Design review of the part built by this model. Coordinates are the model's own, in mm. A direction names the side the tool comes from. Give positions to 0.01 mm unless a question says otherwise; leave off trailing zeros. Write each loop counter-clockwise with the first axis right and the second up, starting at its lowest first coordinate (ties: lowest second). Pieces come first, ordered by that corner, then holes. Notation, with made-up numbers: M 3.25,77 L 33.25,77 A14 ccw 33.25,101 Z; hole C -18,-2 d1. An arc over 180 degrees is marked long. Answer in a Markdown table with one row per item.
```python
from build123d import *

# Parameters (mm, degrees)
SKETCH001_W                 = 93
SKETCH001_H                 = 73
PAD_DEPTH                   = 10
THICKNESS_T                 = 2.5
SKETCH002_R                 = 1.7
HOLE_DEPTH                  = 25
SKETCH003_R                 = 3.7
SKETCH003_R_2               = 1.7
PAD001_DEPTH                = 2
SKETCH003_MIRRORED_2_R      = 3.7
SKETCH003_MIRRORED_2_R_2    = 1.7
PAD001_MIRRORED_2_DEPTH     = 2
SKETCH005_R                 = 1.7
POCKET_DEPTH                = 254.24889
SKETCH005_MIRRORED004_2_R   = 1.7
POCKET_MIRRORED004_2_DEPTH  = 254.24889
SKETCH006_R                 = 3.2
SKETCH006_R_2               = 2.7
PAD003_DEPTH                = 2
SKETCH006_MIRRORED006_2_R   = 3.2
SKETCH006_MIRRORED006_2_R_2 = 2.7
PAD003_MIRRORED006_2_DEPTH  = 2


with BuildPart() as part:
    # Sketch001 → Pad (new body)
    with BuildSketch(Plane.XY):
        Rectangle(SKETCH001_W, SKETCH001_H)
    extrude(amount=PAD_DEPTH)

    # Thickness
    thickness_openings = [part.faces().sort_by_distance(p)[0] for p in [
        (0, 0, 10),
    ]]
    offset(amount=THICKNESS_T, openings=thickness_openings)

    # Sketch002 → Hole (cut)
    with BuildSketch(Plane.XY):
        with Locations((-40, 30)):
            Circle(SKETCH002_R)
    extrude(amount=-HOLE_DEPTH, mode=Mode.SUBTRACT)

    # Sketch003 → Pad001 (join)
    with BuildSketch(Plane.XY):
        with Locations((-40, 30)):
            Circle(SKETCH003_R)
        with Locations((-40, 30)):
            Circle(SKETCH003_R_2, mode=Mode.SUBTRACT)
    pad001 = extrude(amount=PAD001_DEPTH)

    # Sketch003 Mirrored 2 → Pad001 Mirrored 2 (add)
    with BuildSketch(Plane(origin=(0, 0, 0), x_dir=(-1, 0, 0), z_dir=(0, 0, -1))):
        with Locations((-40, 30)):
            Circle(SKETCH003_MIRRORED_2_R)
        with Locations((-40, 30)):
            Circle(SKETCH003_MIRRORED_2_R_2, mode=Mode.SUBTRACT)
    pad001_mirrored_2 = extrude(amount=-PAD001_MIRRORED_2_DEPTH)

    # Mirrored001: Pad001, Pad001 Mirrored 2 across Sketch003 H_Axis
    add(pad001.mirror(Plane.ZX))
    add(pad001_mirrored_2.mirror(Plane.ZX))

    # Sketch005 → Pocket (cut, through all)
    with BuildSketch(Plane.XY):
        with Locations((-40, 30)):
            Circle(SKETCH005_R)
    pocket = extrude(amount=-POCKET_DEPTH, mode=Mode.SUBTRACT)

    # Sketch005 Mirrored004 2 → Pocket Mirrored004 2 (cut, through all)
    with BuildSketch(Plane(origin=(0, 0, 0), x_dir=(-1, 0, 0), z_dir=(0, 0, -1))):
        with Locations((-40, 30)):
            Circle(SKETCH005_MIRRORED004_2_R)
    pocket_mirrored004_2 = extrude(amount=POCKET_MIRRORED004_2_DEPTH, mode=Mode.SUBTRACT)

    # Mirrored005: Pocket, Pocket Mirrored004 2 across Sketch005 H_Axis
    add(pocket.mirror(Plane.ZX), mode=Mode.SUBTRACT)
    add(pocket_mirrored004_2.mirror(Plane.ZX), mode=Mode.SUBTRACT)

    # Sketch006 (on Face35 of MultiTransform002) → Pad003 (join)
    with BuildSketch(Plane(origin=(0, 0, -2.5), x_dir=(1, 0, 0), z_dir=(0, 0, -1))):
        with Locations((-40, 30)):
            Circle(SKETCH006_R)
        with Locations((-40, 30)):
            Circle(SKETCH006_R_2, mode=Mode.SUBTRACT)
    pad003 = extrude(amount=PAD003_DEPTH)

    # Sketch006 Mirrored006 2 → Pad003 Mirrored006 2 (add)
    with BuildSketch(Plane(origin=(0, 0, -2.5), x_dir=(-1, 0, 0), z_dir=(0, 0, 1))):
        with Locations((-40, 30)):
            Circle(SKETCH006_MIRRORED006_2_R)
        with Locations((-40, 30)):
            Circle(SKETCH006_MIRRORED006_2_R_2, mode=Mode.SUBTRACT)
    pad003_mirrored006_2 = extrude(amount=-PAD003_MIRRORED006_2_DEPTH)

    # Mirrored007: Pad003, Pad003 Mirrored006 2 across Sketch006 H_Axis
    add(pad003.mirror(Plane(origin=(0, 0, -2.5), x_dir=(0, 0, -1), z_dir=(0, -1, 0))))
    add(pad003_mirrored006_2.mirror(Plane(origin=(0, 0, -2.5), x_dir=(0, 0, -1), z_dir=(0, -1, 0))))


solid = part.part
```
1) To check wall thickness, follow probe 1 along X at (y, z) = (-30, -3.45); probe 2 along Y at (x, z) = (40, 1.2); probe 3 along Y at (x, z) = (-40, -3.1). State the ranges of each line that lie inside material, in increasing order. Write a range as [from, to].
Geometry says:
| item | result |
|---|---|
| probe 1 | [-43.2, -42.7], [-37.3, -36.8], [36.8, 37.3], [42.7, 43.2] |
| probe 2 | [-39, -36.5], [-33.7, -31.7], [-28.3, -26.3], [26.3, 28.3], [31.7, 33.7], [36.5, 39] |
| probe 3 | [-33.2, -32.7], [-27.3, -26.8], [26.8, 27.3], [32.7, 33.2] |
2) Add section A-A (z = 5.5). Write out the cut boundary in (x, y), and give its area (3 significant figures).
Geometry says:
| item | result |
|---|---|
| outline | M -49,-36.5 A2.5 ccw -46.5,-39 L 46.5,-39 A2.5 ccw 49,-36.5 L 49,36.5 A2.5 ccw 46.5,39 L -46.5,39 A2.5 ccw -49,36.5 Z; hole M -46.5,-36.5 L 46.5,-36.5 L 46.5,36.5 L -46.5,36.5 Z |
| area | 850 mm^2 |
3) Insertion check: P1, Ø3, axis at x = 40, y = -30, coming from the +Z side; P2, Ø6, axis at x = 38.5, y = 31, coming from the +Z side; P3, Ø1.5, axis at x = -36.5, y = 3.5, coming from the +Z side; P4, Ø5, axis at x = 12, y = -14, coming from the -Z side. Each pin has a flat end and moves straight along its axis. Give the tip position at first contact, or say it passes through.
Geometry says:
| item | result |
|---|---|
| P1 | through |
| P2 | z = 2 |
| P3 | z = 0 |
| P4 | z = -2.5 |
4) Add section B-B (y = 30). Count the separate pieces of the cut face and the enclosed holes in it, and give its area (3 significant figures).
Geometry says:
| item | result |
|---|---|
| separate pieces | 3 |
| enclosed holes | 0 |
| area | 295 mm^2 |
5) For faces 5 (the face through (42.73, -32.5, 0.99)), 6 (the face through (-1, 39, 5)), 7 (the face through (40, 28, -2.5)), list the 3-axis set-ups (+Z, -Z, +X, -X, +Y, -Y) from which the entire face can be reached by the end or side of a thin tool; tool diameter is ignored.
Geometry says:
| item | result |
|---|---|
| face 5 | +Z |
| face 6 | +Z, -Z, +X, -X, +Y |
| face 7 | -Z |
6) Add section C-C (x = 18.5). Write out the cut boundary in (y, z).
Geometry says:
| item | result |
|---|---|
| outline | M -39,0 A2.5 ccw -36.5,-2.5 L 36.5,-2.5 A2.5 ccw 39,0 L 39,10 L 36.5,10 L 36.5,0 L -36.5,0 L -36.5,10 L -39,10 Z |
7) The part is to be moulded in two halves that separate along X. For faces 1 (the face through (-48.287, 38.248, 5.07)), 2 (the face through (48, 1, -2)), 3 (the face through (40, -32, -2.5)), 4 (the face through (1, -38, -2)), say which applies: released by +X, released by -X, zero draft, split by the parting line, or undercut.
Geometry says:
| item | result |
|---|---|
| face 1 | released by -X |
| face 2 | released by +X |
| face 3 | undercut |
| face 4 | zero draft |
8) Add section D-D (y = -21). Write out the cut boundary in (x, z), and give its area (3 significant figures).
Geometry says:
| item | result |
|---|---|
| outline | M -49,0 A2.5 ccw -46.5,-2.5 L 46.5,-2.5 A2.5 ccw 49,0 L 49,10 L 46.5,10 L 46.5,0 L -46.5,0 L -46.5,10 L -49,10 Z |
| area | 292 mm^2 |
